Source: three-view drawing plus pictorial views. Frame: mm from the lowest corner of the part. A direction names the side the tool comes from. Round coordinates to 2 decimals unless told otherwise and drop trailing zeros. Loops run counter-clockwise (first coordinate to the right, second up) from the corner with the lowest first, then second, coordinate; pieces in that order, holes last. Notation, with made-up numbers: M 76.5,81 L 95.5,81 A19 cw 95.5,108 Z; hole C 67,36.25 d6. An arc over 180 degrees is marked long. Return JSON: item names as keys, results as strings. Group by question number.
1) Material intervals for line 1 (Y direction, x = 10, z = 26); line 2 (Y direction, x = 10, z = 30) (1 decimal); line 3 (Z direction, x = 38.5, y = 21.5) (1 decimal), sorted ascending. Write a range as from..to.
2) Access query for the marked faces 4 and 5. Directions: +Z, -Z, +X, -X, +Y, -Y. A direction counts if a zero-diameter tool reaches every point of the face in a straight line with its end or side. Return the directions, or none.
3) Contact query for flat-ended pins moving along their axis: P1, Ø7, axis at x = 30, y = 30, coming from the -Z side; P2, Ø10, axis at y = 35, z = 20.5, coming from the +X side (1 decimal); P3, Ø3, axis at x = 31.5, y = 30, coming from the +Z side. Output: stop coordinate, or through.
4) Section D-D (z = 9.5). Output: boundary loops of the cut face in (x, y) (1 decimal).
5) Section C-C (x = 18.5). Output: boundary loops of the cut face in (y, z) (1 decimal), plus the area to 3 significant figures.
6) Mould query, pull axis X, two halves, no side actions, for the marked faces 1, 2 and 3. Classes: +X half, -X half, draft (parallel to the pull), parting line (faces both ways), or undercut.
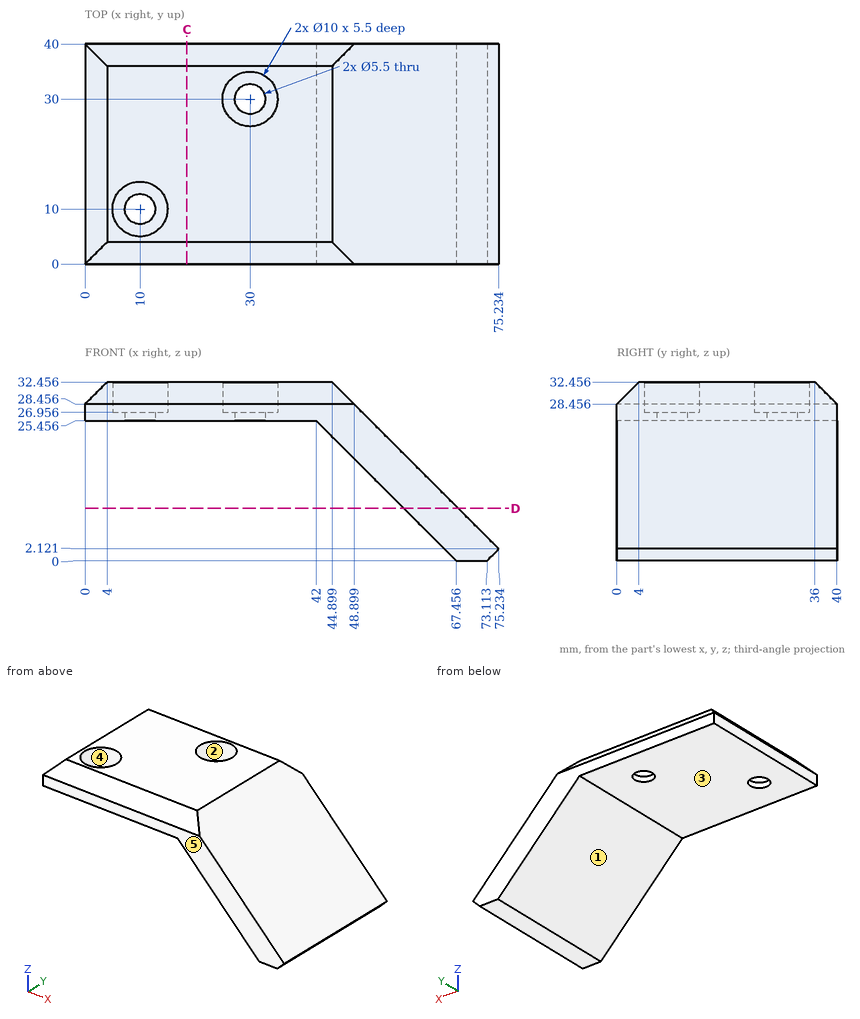
Returned:
{
 "1": {"line 1": "y = 0..7.25, 12.75..40", "line 2": "y = 1.5..5, 15..38.5", "line 3": "z = 25.5..32.5"},
 "2": {"face 4": "+Z", "face 5": "+Z, -Z, +X, -X, -Y"},
 "3": {"P1": "stops at z = 25.46", "P2": "stops at x = 61.9", "P3": "stops at z = 26.96"},
 "4": {"outline": "M 58,0 L 67.9,0 L 67.9,40 L 58,40 Z"},
 "5": {"outline": "M 0,25.5 L 40,25.5 L 40,28.5 L 36,32.5 L 4,32.5 L 0,28.5 Z", "area": "264 mm^2"},
 "6": {"face 1": "-X half", "face 2": "undercut", "face 3": "draft"}
}
